Check sheet for the modelled part. Datum: model origin and axes. Units: mm. Round coordinates to 2 decimals unless told otherwise and drop trailing zeros. Write each loop counter-clockwise with the first axis right and the second up, starting at its lowest first coordinate (ties: lowest second). Pieces come first, ordered by that corner, then holes. Notation, with made-up numbers: (-24.75, 68.5) -> (25.25, 68.5) arc R22 cw to (25.25, 82.5) -> close; hole circle Ø7 at (-36, -26.75). An arc over 180 degrees is marked (long way). One line per item, written item: value. Start each with the question number.
```python
from build123d import *

# Parameters (mm, degrees)
SKETCH1_R           = 2.0828
BOSS_EXTRUDE1_DEPTH = 18.542


with BuildPart() as part:
    # Sketch1 → Boss-Extrude1 (new body)
    with BuildSketch(Plane.XY):
        with BuildLine():
            Line((-2.54, 0), (-2.54, 27.94))
            ThreePointArc((-2.54, 27.94), (-2.289263959, 29.040395622), (-1.586558642, 29.923540188))
            Line((-1.586558642, 29.923540188), (11.083668211, 40.057974582))
            ThreePointArc((11.083668211, 40.057974582), (16.002, 41.783), (20.920331789, 40.057974582))
            Line((20.920331789, 40.057974582), (33.590558642, 29.923540188))
            ThreePointArc((33.590558642, 29.923540188), (34.293263959, 29.040395622), (34.544, 27.94))
            Line((34.544, 27.94), (34.544, 0))
            ThreePointArc((34.544, 0), (34.293263959, -1.100395622), (33.590558642, -1.983540188))
            Line((33.590558642, -1.983540188), (20.920331789, -12.117974582))
            ThreePointArc((20.920331789, -12.117974582), (16.002, -13.843), (11.083668211, -12.117974582))
            Line((11.083668211, -12.117974582), (-1.586558642, -1.983540188))
            ThreePointArc((-1.586558642, -1.983540188), (-2.289263959, -1.100395622), (-2.54, 0))
        make_face()
        with Locations((16.002, 33.909)):
            Circle(SKETCH1_R, mode=Mode.SUBTRACT)
        with Locations((16.002, -5.969)):
            Circle(SKETCH1_R, mode=Mode.SUBTRACT)
    extrude(amount=BOSS_EXTRUDE1_DEPTH)


solid = part.part
```
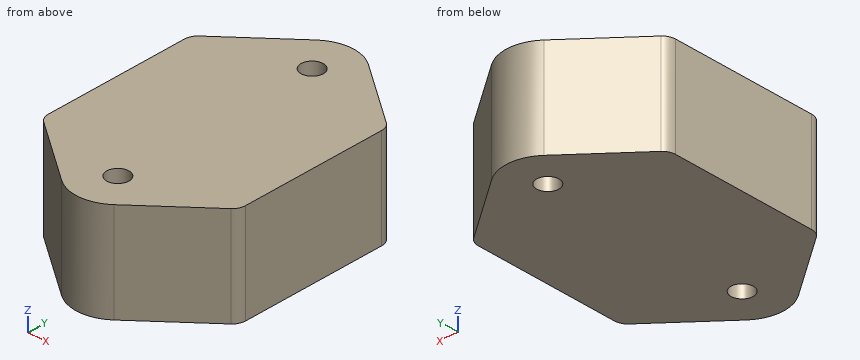
1. Cross-section at C-C (x = 2). Record the cut outline in (y, z).
2. Material ranges on probe 1 along Y at (x, z) = (16, 8.25); probe 2 along Y at (x, z) = (14.5, 2.25); probe 3 along Y at (x, z) = (26, 4.5), recorded low to high.
3. Cross-section at D-D (y = 37). Record the cut outline in (x, z), plus the area to 3 significant figures.
4. Cross-section at B-B (x = 15.5). Record the cut outline in (y, z).
5. Depth check by flat-ended pin: pin 1 Ø3.5 at (x, y) = (16.002, -5.969) entering from +Z; pin 2 Ø1 at (y, z) = (-1, 6.5) entering from -X; pin 3 Ø1.5 at (x, z) = (9.5, 5.5) entering from +Y. Enter the tip coordinate at first touch or a pass-through.
6. Cross-section at A-A (z = 17.25). Record the cut outline in (x, y).
Working result:
1. outline: (-4.85, 0) -> (32.79, 0) -> (32.79, 18.54) -> (-4.85, 18.54) -> close
2. probe 1: y = -13.84 to -8.05, -3.89 to 31.83, 35.99 to 41.78
2. probe 2: y = -13.7 to -7.41, -4.53 to 32.47, 35.35 to 41.64
2. probe 3: y = -8.05 to 35.99
3. outline: (7.26, 0) -> (24.74, 0) -> (24.74, 18.54) -> (7.26, 18.54) -> close
3. area: 324 mm^2
4. outline: (-13.83, 0) -> (-7.99, 0) -> (-7.99, 18.54) -> (-13.83, 18.54) -> close; (-3.95, 0) -> (31.89, 0) -> (31.89, 18.54) -> (-3.95, 18.54) -> close; (35.93, 0) -> (41.77, 0) -> (41.77, 18.54) -> (35.93, 18.54) -> close
5. pin 1: passes through
5. pin 2: stops at x = -2.49
5. pin 3: stops at y = 39.39
6. outline: (-2.54, 0) arc R2.54 ccw to (-1.59, -1.98) -> (11.08, -12.12) arc R7.87 ccw to (20.92, -12.12) -> (33.59, -1.98) arc R2.54 ccw to (34.54, 0) -> (34.54, 27.94) arc R2.54 ccw to (33.59, 29.92) -> (20.92, 40.06) arc R7.87 ccw to (11.08, 40.06) -> (-1.59, 29.92) arc R2.54 ccw to (-2.54, 27.94) -> close; hole circle Ø4.17 at (16, -5.97); hole circle Ø4.17 at (16, 33.91)
